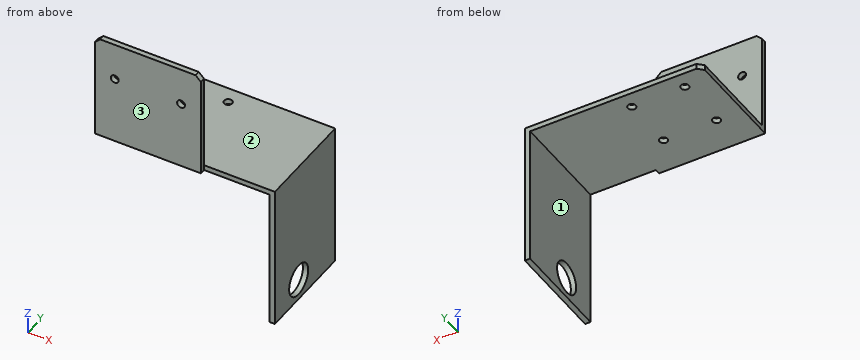
from build123d import *

# Parameters (mm, degrees)
EXTRUDE1_DEPTH           = 40
EXTRUDE2_REACH           = 42
SKETCH2_R                = 1.5
EXTRUDE3_REACH           = 42
SKETCH3_R                = 1.5
CHAMFER1_SIZE            = 2
SKETCH4_W                = 2
SKETCH4_H                = 38
BOSS_EXTRUDE1_DEPTH      = 26.69
BOSS_EXTRUDE1_DEPTH_BACK = 3
SKETCH5_W                = 53
SKETCH5_H                = 38
BOSS_EXTRUDE2_DEPTH      = 2
SKETCH6_R                = 6
CUT_EXTRUDE1_DEPTH       = 3


with BuildPart() as part:
    # Sketch1 → Extrude1 (new body)
    with BuildSketch(Plane(origin=(0, 0, 0), x_dir=(0, 0, -1), z_dir=(1, 0, 0))):
        Polygon((0, 0), (0, 38), (2, 38), (2, -2), (-38, -2), (-38, 0), align=None)
    extrude(amount=EXTRUDE1_DEPTH)

    # Sketch2 → Extrude2 (cut, up to next)
    with BuildSketch(Plane(origin=(0, -2, 0), x_dir=(-1, 0, 0), z_dir=(0, -1, 0)), mode=Mode.PRIVATE) as extrude2_sk1:
        with Locations((-32.5, -23.75)):
            Circle(SKETCH2_R)
    extrude2_tool1 = extrude(extrude2_sk1.sketch, amount=-EXTRUDE2_REACH, mode=Mode.PRIVATE) & part.part
    add(extrude2_tool1.solids().sort_by_distance((32.5, -2, 23.75))[0], mode=Mode.SUBTRACT)
    # Sketch2 → Extrude2 (cut, up to next)
    with BuildSketch(Plane(origin=(0, -2, 0), x_dir=(-1, 0, 0), z_dir=(0, -1, 0)), mode=Mode.PRIVATE) as extrude2_sk2:
        with Locations((-7.5, -23.75)):
            Circle(SKETCH2_R)
    extrude2_tool2 = extrude(extrude2_sk2.sketch, amount=-EXTRUDE2_REACH, mode=Mode.PRIVATE) & part.part
    add(extrude2_tool2.solids().sort_by_distance((7.5, -2, 23.75))[0], mode=Mode.SUBTRACT)

    # Sketch3 → Extrude3 (cut, up to next)
    with BuildSketch(Plane(origin=(0, 0, -2), x_dir=(-1, 0, 0), z_dir=(0, 0, -1)), mode=Mode.PRIVATE) as extrude3_sk1:
        with Locations((-10, 31.9)):
            Circle(SKETCH3_R)
    extrude3_tool1 = extrude(extrude3_sk1.sketch, amount=-EXTRUDE3_REACH, mode=Mode.PRIVATE) & part.part
    add(extrude3_tool1.solids().sort_by_distance((10, 31.9, -2))[0], mode=Mode.SUBTRACT)
    # Sketch3 → Extrude3 (cut, up to next)
    with BuildSketch(Plane(origin=(0, 0, -2), x_dir=(-1, 0, 0), z_dir=(0, 0, -1)), mode=Mode.PRIVATE) as extrude3_sk2:
        with Locations((-30, 31.9)):
            Circle(SKETCH3_R)
    extrude3_tool2 = extrude(extrude3_sk2.sketch, amount=-EXTRUDE3_REACH, mode=Mode.PRIVATE) & part.part
    add(extrude3_tool2.solids().sort_by_distance((30, 31.9, -2))[0], mode=Mode.SUBTRACT)
    # Sketch3 → Extrude3 (cut, up to next)
    with BuildSketch(Plane(origin=(0, 0, -2), x_dir=(-1, 0, 0), z_dir=(0, 0, -1)), mode=Mode.PRIVATE) as extrude3_sk3:
        with Locations((-30, 11.9)):
            Circle(SKETCH3_R)
    extrude3_tool3 = extrude(extrude3_sk3.sketch, amount=-EXTRUDE3_REACH, mode=Mode.PRIVATE) & part.part
    add(extrude3_tool3.solids().sort_by_distance((30, 11.9, -2))[0], mode=Mode.SUBTRACT)
    # Sketch3 → Extrude3 (cut, up to next)
    with BuildSketch(Plane(origin=(0, 0, -2), x_dir=(-1, 0, 0), z_dir=(0, 0, -1)), mode=Mode.PRIVATE) as extrude3_sk4:
        with Locations((-10, 11.9)):
            Circle(SKETCH3_R)
    extrude3_tool4 = extrude(extrude3_sk4.sketch, amount=-EXTRUDE3_REACH, mode=Mode.PRIVATE) & part.part
    add(extrude3_tool4.solids().sort_by_distance((10, 11.9, -2))[0], mode=Mode.SUBTRACT)

    # Chamfer1
    chamfer1_edges = [part.edges().sort_by_distance(p)[0] for p in [
        (40, 38, -1),
        (0, 38, -1),
        (40, -1, 38),
        (0, -1, 38),
    ]]
    chamfer(chamfer1_edges, length=CHAMFER1_SIZE)

    # Sketch4 → Boss-Extrude1 (add, two sides)
    with BuildSketch(Plane(origin=(40, 0, 0), x_dir=(0, 0, -1), z_dir=(1, 0, 0))) as boss_extrude1_sk:
        with Locations((1, 19)):
            Rectangle(SKETCH4_W, SKETCH4_H)
    extrude(amount=BOSS_EXTRUDE1_DEPTH)
    extrude(boss_extrude1_sk.sketch, amount=-BOSS_EXTRUDE1_DEPTH_BACK)

    # Sketch5 → Boss-Extrude2 (add)
    with BuildSketch(Plane(origin=(66.69, 0, 0), x_dir=(0, 0, -1), z_dir=(1, 0, 0))):
        with Locations((28.5, 19)):
            Rectangle(SKETCH5_W, SKETCH5_H)
    extrude(amount=-BOSS_EXTRUDE2_DEPTH)

    # Sketch6 → Cut-Extrude1 (cut)
    with BuildSketch(Plane(origin=(66.69, 0, 0), x_dir=(0, 0, -1), z_dir=(1, 0, 0))):
        with Locations((47, 15)):
            Circle(SKETCH6_R)
    extrude(amount=-CUT_EXTRUDE1_DEPTH, mode=Mode.SUBTRACT)


solid = part.part
Can you work these out from the model? Positions are in its coordinate system, mm. Face numbers are marked on the shaded views. A direction names the side the tool comes from. Round coordinates to 2 decimals unless told otherwise and drop trailing zeros. Loops run counter-clockwise (first coordinate to the right, second up) from the corner with the lowest first, then second, coordinate; pieces in that order, holes last. Notation, with made-up numbers: (13, -21) - (51, -21) arc R20 ccw to (51, -14) - close; hole circle Ø5 at (17, -4.5). An arc over 180 degrees is marked (long way). Answer in a Markdown table with one row per item. Add a question column.
Q1. Which directions (+Z, -Z, +X, -X, +Y, -Y) give clear straight access to the entire face, cutting with the end or side of a thin tool? Please do the marked faces 1, 2 and 3.
Q2. I want a section at C-C on z = -49. List the corners of the cut face in (x, y) for me, and give its area (3 significant figures).
Q3. I need wall thicknesses on L1, parallel to X at y = -0.6, z = 23.75; L2, parallel to Y at x = 30, z = -0.45; L3, parallel to X at y = -1, z = 23. Which ranges of each line are inside material? Lowest first, please.
Q4. I want a section at B-B on x = 10. List the corners of the cut face in (y, z) for me, and give its area (3 significant figures).
Q5. For pin 1 Ø8 at (y, z) = (6, 8) entering from +X; pin 2 Ø19 at (x, y) = (28.5, 18.5) entering from +Z; pin 3 Ø19 at (y, z) = (21, -38.5) entering from -X; pin 4 Ø2 at (x, z) = (32, 16.5) entering from +Y, each with a flat end and sliding along its axis, tell me the tip position at first contact or that it passes through.
Q6. I want a section at D-D on y = 15. List the corners of the cut face in (x, z) for me, and give its area (3 significant figures).
Q7. I want a section at A-A on y = 31.9. List the corners of the cut face in (x, z) for me, and give its area (3 significant figures).
A:
| question | item | result |
|---|---|---|
| 1 | face 1 | -Z, -X, +Y, -Y |
| 1 | face 2 | +Z, +X, -X, +Y |
| 1 | face 3 | +Z, -Z, +X, -X, -Y |
| 2 | outline | (64.69, 0) - (66.69, 0) - (66.69, 9.34) - (64.69, 9.34) - close; (64.69, 20.66) - (66.69, 20.66) - (66.69, 38) - (64.69, 38) - close |
| 2 | area | 53.4 mm^2 |
| 3 | L1 | 0 to 6, 9 to 31, 34 to 40 |
| 3 | L2 | -2 to 10.4, 13.4 to 30.4, 33.4 to 38 |
| 3 | L3 | 0 to 6.2, 8.8 to 31.2, 33.8 to 40 |
| 4 | outline | (-2, -2) - (10.4, -2) - (10.4, 0) - (0, 0) - (0, 38) - (-2, 38) - close; (13.4, -2) - (30.4, -2) - (30.4, 0) - (13.4, 0) - close; (33.4, -2) - (38, -2) - (38, 0) - (33.4, 0) - close |
| 4 | area | 144 mm^2 |
| 5 | pin 1 | through |
| 5 | pin 2 | z = 0 |
| 5 | pin 3 | x = 64.69 |
| 5 | pin 4 | y = 0 |
| 6 | outline | (0, -2) - (64.69, -2) - (64.69, -41) - (66.69, -41) - (66.69, 0) - (0, 0) - close; (64.69, -55) - (66.69, -55) - (66.69, -53) - (64.69, -53) - close |
| 6 | area | 215 mm^2 |
| 7 | outline | (0, -2) - (8.5, -2) - (8.5, 0) - (0, 0) - close; (11.5, -2) - (28.5, -2) - (28.5, 0) - (11.5, 0) - close; (31.5, -2) - (64.69, -2) - (64.69, -55) - (66.69, -55) - (66.69, 0) - (31.5, 0) - close |
| 7 | area | 227 mm^2 |
